Geometry: final body of the model. Coordinates: model frame, mm. A direction names the side the tool comes from. Give positions to 0.01 mm unless a question says otherwise; leave off trailing zeros. Loops run counter-clockwise (first coordinate to the right, second up) from the corner with the lowest first, then second, coordinate; pieces in that order, holes last. Notation, with made-up numbers: (16, 50) - (68, 50) arc R13 ccw to (68, 72) - close; hole circle Ø7 at (42, 89). An arc over 180 degrees is marked (long way). Use CSV: the item, a comma, the result in double quotes. Start each with the question number.
Autodesk Inventor part; units mm, degrees
ref_plane "YZ Plane" through (0, 0, 0) normal (1, 0, 0) x (0, 1, 0)
ref_plane "XZ Plane" through (0, 0, 0) normal (0, 1, 0) x (-1, 0, 0)
ref_plane "XY Plane" through (0, 0, 0) normal (0, 0, 1) x (1, 0, 0)
sketch "Sketch1" plane through (0, 0, 0) normal (0, 1, 0) x (-1, 0, 0)
  line L0 (0, 0) -> (34.038, 0)
  line L1 (34.038, 0) -> (34.038, -150)
  line L2 (34.038, -150) -> (0, -150)
  line L3 (0, -150) -> (0, 0)
  line L4 (0, 0) -> (-5, 0)
  line L5 (-5, 0) -> (-5, -150)
  line L6 (-5, -150) -> (0, -150)
  dimension "d0" = 34.038
  dimension "d1" = 150
  dimension "d2" = 5
extrude "Extrusion1" add sketch "Sketch1" along normal blind 4 contours L0 L1 L2 L3
extrude "Extrusion2" add sketch "Sketch1" along normal blind 2 contours L3 L6 L5 L4
chamfer "Chamfer1" distance 4 angle 45 1 edges at (-34.038, 4, -75)
properties part number "frontWallipt"
Item 1: Section B-B (y = 2.95). Output: boundary loops of the cut face in (x, z).
Item 2: Ray query, probe 1 along X at (y, z) = (2.05, -130.5); probe 2 along X at (y, z) = (0.3, -109). Return the intervals inside material, ascending.
Item 3: Reachability of faces 1 (the flat face through (3, 2, -74)), 2 (the flat face through (-32.01, 2.03, -76.05)) from +Z, -Z, +X, -X, +Y, -Y: full face, straight path, thin tool, end or side. Return the list, or none.
Item 4: Pin query (flat end, axial travel): pin 1 Ø2 at (y, z) = (2.5, -52.5) entering from +X. Return the tip coordinate at first contact, or that it passes through.
Outcome:
1,outline,"(-31.09, -150) - (0, -150) - (0, 0) - (-31.09, 0) - close"
2,probe 1,"x = -31.99 to 0"
2,probe 2,"x = -33.74 to 5"
3,face 1,"+Z, -Z, +X, +Y"
3,face 2,"+Z, -Z, -X, +Y"
4,pin 1,"stops at x = 5"
